Verification items for the finished model (mm, model axes). Face numbers are marked on the shaded views. Round coordinates to 2 decimals unless told otherwise and drop trailing zeros. Order: outer loops, then holes, each group sorted by start corner. A loop starts at its lowest first (then second) coordinate and runs counter-clockwise, first axis right, second up. Notation, with made-up numbers: (19.25, -7) -> (67.25, -7) arc R23 cw to (67.25, 22) -> close; hole circle Ø1 at (-38, 21.5). An arc over 180 degrees is marked (long way). Put each result on its own line as item: value.
from build123d import *

# Parameters (mm, degrees)
SKETCH1_W                     = 6
SKETCH1_H                     = 6
SKETCH1_R                     = 1.5
BOSS_EXTRUDE1_DEPTH           = 8
CSK_FOR_M3_SFHCS1_D           = 3.4
CSK_FOR_M3_SFHCS1_DEPTH       = 11.3
CSK_FOR_M3_SFHCS1_CSINK_D     = 6.72
CSK_FOR_M3_SFHCS1_CSINK_ANGLE = 90
CSK_FOR_M3_SFHCS1_TIP         = 1.021463052


with BuildPart() as part:
    # Sketch1 → Boss-Extrude1 (new body)
    with BuildSketch(Plane(origin=(0, 0, 0), x_dir=(1, 0, 0), z_dir=(0, 1, 0))):
        Rectangle(SKETCH1_W, SKETCH1_H)
        with Locations(Location((0, 0, 0), (0, 0, 270))):
            Circle(SKETCH1_R, mode=Mode.SUBTRACT)
    extrude(amount=BOSS_EXTRUDE1_DEPTH)

    # CSK for M3 SFHCS1
    with Locations(Plane(origin=(0, 8, 0), x_dir=(1, 0, 0), z_dir=(0, 1, 0))):
        with Locations((0, 0)):
            CounterSinkHole(CSK_FOR_M3_SFHCS1_D / 2, CSK_FOR_M3_SFHCS1_CSINK_D / 2, depth=CSK_FOR_M3_SFHCS1_DEPTH, counter_sink_angle=CSK_FOR_M3_SFHCS1_CSINK_ANGLE)
            with Locations((0, 0, -(CSK_FOR_M3_SFHCS1_DEPTH + CSK_FOR_M3_SFHCS1_TIP / 2))):  # 118° drill point
                Cone(0, CSK_FOR_M3_SFHCS1_D / 2, CSK_FOR_M3_SFHCS1_TIP, mode=Mode.SUBTRACT)


solid = part.part
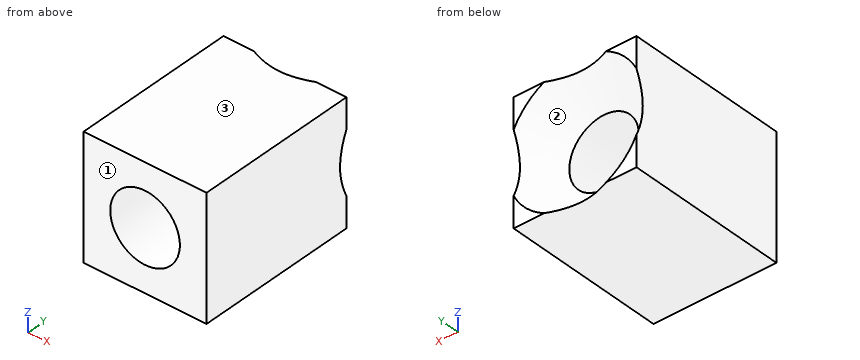
Item 1: Material ranges on L1, parallel to Z at x = 0, y = 1.75; L2, parallel to X at y = 6.25, z = -1, recorded low to high. Write a range as [from, to].
Check sheet entries:
L1: z = [-3, -1.7], [1.7, 3]
L2: x = [-3, -1.37], [1.37, 3]
Item 2: Release check for a two-part mould opening along Z. For the marked faces 1, 2 and 3 record: +Z half, -Z half, draft (parallel to the pull), parting line (faces both ways), or undercut.
Check sheet entries:
face 1: draft
face 2: undercut
face 3: +Z half
Item 3: Section check C-C on y = 5.5. Record the boundary of the cut face in (x, z).
Check sheet entries:
outline: (-3, -3) -> (3, -3) -> (3, 3) -> (-3, 3) -> close; hole circle Ø3.4 at (0, 0)
Item 4: Section check A-A on x = 0. Record the boundary of the cut face in (y, z), then the cut area to 3 significant figures.
Check sheet entries:
outline: (0, -3) -> (7.64, -3) -> (6.34, -1.7) -> (0, -1.7) -> close; (0, 1.7) -> (6.34, 1.7) -> (7.64, 3) -> (0, 3) -> close
area: 18.2 mm^2
Item 5: Gauge pin test, flat ends, axial feed: pin 1 Ø1 at (x, z) = (1.5, -2) entering from -Y; pin 2 Ø2 at (x, z) = (-0.5, -1) entering from +Y. Record the tip position at first contact, or that the pin passes through.
Check sheet entries:
pin 1: stops at y = 0
pin 2: stops at y = 6.76
Item 6: Section check B-B on z = 0. Record the boundary of the cut face in (x, y), then the cut area to 3 significant figures.
Check sheet entries:
outline: (-3, 0) -> (-1.7, 0) -> (-1.7, 6.34) -> (-3, 7.64) -> close; (1.7, 0) -> (3, 0) -> (3, 7.64) -> (1.7, 6.34) -> close
area: 18.2 mm^2
